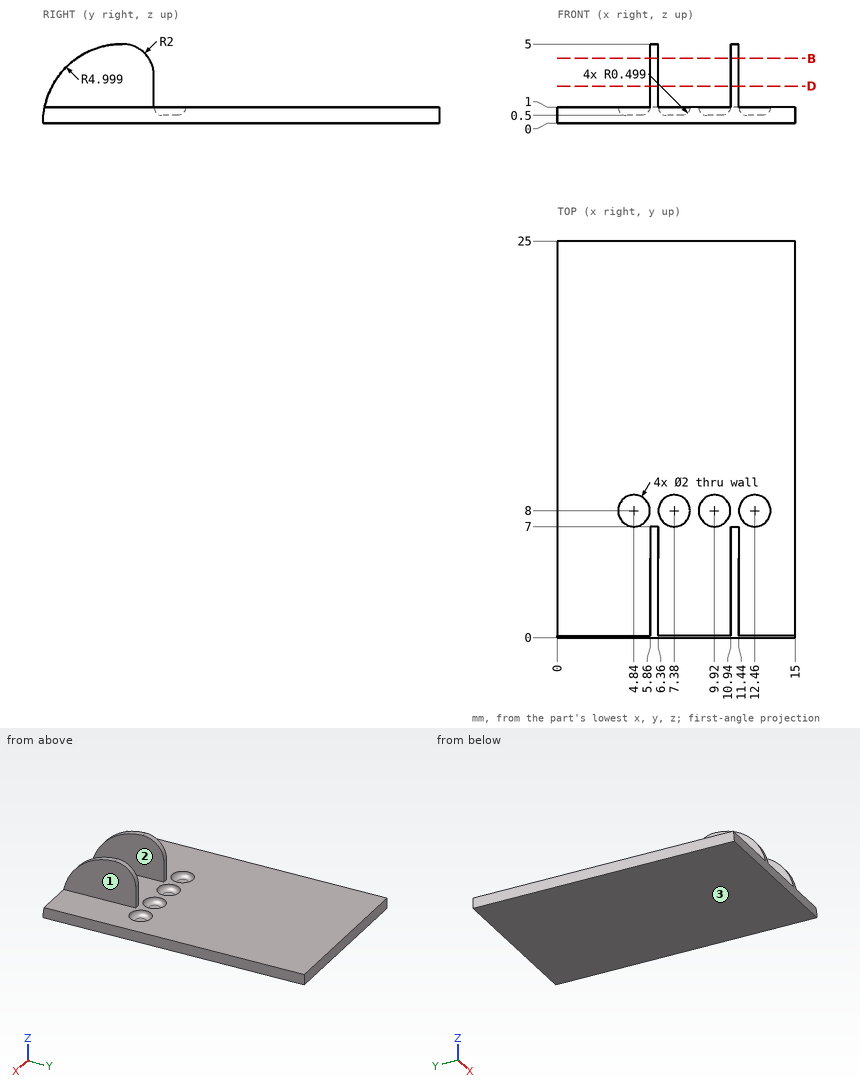
For this review, use the dimensioned drawing (mm, ordinates from the lowest corner) and the shaded views. Give positions to 0.01 mm unless a question says otherwise; leave off trailing zeros. Order: outer loops, then holes, each group sorted by start corner. A loop starts at its lowest first (then second) coordinate and runs counter-clockwise, first axis right, second up. Notation, with made-up numbers: (-26.75, 68) - (20.25, 68) arc R12 cw to (20.25, 80) - close; hole circle Ø7 at (30.25, 5.5). An arc over 180 degrees is marked (long way). Use CSV: the item, a comma, the result in double quotes. Start each with the question number.
Q1. To check wall thickness, follow line 1 along X through (y, z) = (4.5, 1.65); line 2 along Z through (x, y) = (7, 20.75); line 3 along Y through (x, z) = (10.75, 0.85) (1 decimal). State the ranges of each line that lie inside material, in increasing order. Write a range as [from, to].
Q2. We need section D-D, the plane z = 2.35. Write out the cut boundary in (x, y).
Q3. We need section B-B, the plane z = 4.1. Write out the cut boundary in (x, y).
Q4. Clearance check with flat-ended pins moving along their axes: pin 1 Ø1.5 at (x, z) = (10.5, 3) entering from -Y; pin 2 Ø2 at (y, z) = (2.5, 2.5) entering from +X; pin 3 Ø0.5 at (x, y) = (10, 8) entering from +Z. State where each tip first meets the part, or that it passes through.
Q5. The part is to be moulded in two halves that separate along X. For the marked faces 1, 2 and 3, say which applies: +X half, -X half, draft (parallel to the pull), parting line (faces both ways), or undercut.
Outcome:
1,line 1,"x = [5.86, 6.36], [10.94, 11.44]"
1,line 2,"z = [0, 1]"
1,line 3,"y = [0.1, 7.5], [8.5, 25]"
2,outline,"(5.86, 0.59) - (6.36, 0.59) - (6.36, 7) - (5.86, 7) - close; (10.94, 0.59) - (11.44, 0.59) - (11.44, 7) - (10.94, 7) - close"
3,outline,"(5.86, 2.14) - (6.36, 2.14) - (6.36, 6.67) - (5.86, 6.67) - close; (10.94, 2.14) - (11.44, 2.14) - (11.44, 6.67) - (10.94, 6.67) - close"
4,pin 1,"stops at y = 0.61"
4,pin 2,"stops at x = 11.44"
4,pin 3,"stops at z = 0.5"
5,face 1,"+X half"
5,face 2,"undercut"
5,face 3,"draft"
